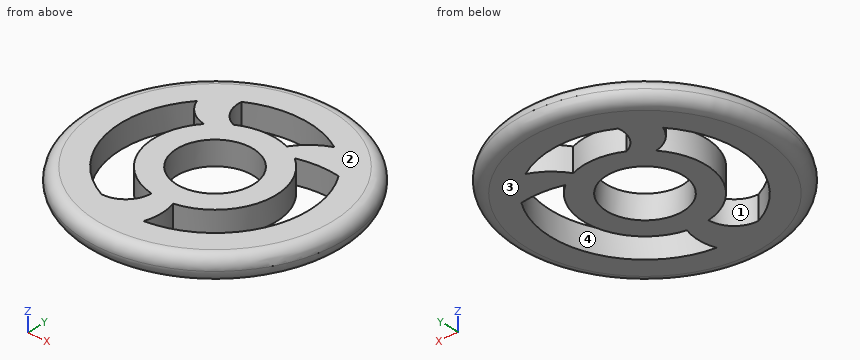
from build123d import *

# Parameters (mm, degrees)
F0_R     = 38.1945033512
F0_R_2   = 11.3
F1_DEPTH = 7
F2_R     = 3.49999


# Not quite as in the source:
# - a fillet or chamfer is up to 0.001 mm smaller than in the source, because OpenCascade refuses the exact size


with BuildPart() as f1:
    # F0 (on Top) → F1 (new body)
    with BuildSketch(Plane.XY):
        Circle(F0_R)
        with BuildLine():
            ThreePointArc((-11.1190587191, -25.3990096631), (-26.9847609568, -6.3691313979), (-21.3025923236, 17.7466255653))
            ThreePointArc((-21.3025923236, 17.7466255653), (-18.3465502514, 13.6852419499), (-13.7577746625, 11.6416763896))
            ThreePointArc((-13.7577746625, 11.6416763896), (-16.9304092047, -6.1778828887), (-3.0268251987, -17.7663536507))
            ThreePointArc((-3.0268251987, -17.7663536507), (-5.4906522747, -23.2602441725), (-11.1190587191, -25.3990096631))
        make_face(mode=Mode.SUBTRACT)
        with BuildLine():
            ThreePointArc((3.3689917925, -27.5207749339), (4.1908869079, -22.6127160748), (3.3689917925, -17.7046572157))
            ThreePointArc((3.3689917925, -17.7046572157), (17.5564618696, -4.0713191283), (10.8174583905, 14.4148391179))
            ThreePointArc((10.8174583905, 14.4148391179), (16.8916900663, 15.5906448864), (23.0748101796, 15.3719320138))
            ThreePointArc((23.0748101796, 15.3719320138), (25.1945379599, -11.5749045633), (3.3689917925, -27.5207749339))
        make_face(mode=Mode.SUBTRACT)
        Circle(F0_R_2, mode=Mode.SUBTRACT)
        with BuildLine():
            ThreePointArc((-8.6949064417, 15.7861836678), (-12.603803519, 19.1055384299), (-13.6713432148, 24.1213086993))
            ThreePointArc((-13.6713432148, 24.1213086993), (0.373914134, 27.7236964866), (14.3169083029, 23.7438264673))
            ThreePointArc((14.3169083029, 23.7438264673), (9.7472249081, 20.9497927504), (6.2279462514, 16.9120571875))
            ThreePointArc((6.2279462514, 16.9120571875), (-1.3558653844, 17.9712721276), (-8.6949064417, 15.7861836678))
        make_face(mode=Mode.SUBTRACT)
    extrude(amount=F1_DEPTH)

    # F2 (radius 3.5 in the source; OpenCascade refuses exactly that, so slightly less here)
    f2_edges = [f1.edges().sort_by_distance(p)[0] for p in [
        (-38.194503, 0, 7),
        (-38.194503, 0, 0),
    ]]
    fillet(f2_edges, radius=F2_R)


solid = f1.part
For this review, take the finished solid that the model builds, in its own axes (mm). Face numbers are marked on the shaded views. A direction names the side the tool comes from. Round coordinates to 2 decimals unless told otherwise and drop trailing zeros. Order: outer loops, then holes, each group sorted by start corner. A loop starts at its lowest first (then second) coordinate and runs counter-clockwise, first axis right, second up. Notation, with made-up numbers: M 77,50 L 114,50 A27 cw 114,85 Z; hole C 63,25 d4. An arc over 180 degrees is marked long. Use a Markdown table: item, result. Add a question column.
Item 1: To check wall thickness, follow line 1 along Y through (x, z) = (-6.5, 5); line 2 along X through (y, z) = (6, 1.75); line 3 along Y through (x, z) = (0, 5.25). State the ranges of each line that lie inside material, in increasing order.
Item 2: Tool access review of the marked faces 1 and 2: name each direction out of +Z, -Z, +X, -X, +Y, -Y from which nothing blocks a thin tool from reaching the whole face with its end or side.
Item 3: Mouldability with a two-part tool opening along Y and no side actions: class the marked faces 3 and 4 as released by +Y, released by -Y, zero draft, split by the parting line, or undercut.
Item 4: Insertion check: pin 1 (2 mm diameter, centred on x = -5, z = 3, fed in from -Y); pin 2 (20.5 mm diameter, centred on x = 0, y = 0, fed in from +Z); pin 3 (4 mm diameter, centred on y = 18.5, z = 3, fed in from +X); pin 4 (1.5 mm diameter, centred on y = 3, z = 3.5, fed in from -X). Each pin has a flat end and moves straight along its axis. Give the tip position at first contact, or say it passes through.
Item 5: Add section A-A, the plane x = 0. State how many separate pieces and enclosed holes the cut face has, then the cut area to 3 significant figures.
Item 6: Add section C-C, the plane z = 5.5. Give the boundary of the cut face in (x, y).
Geometry results:
| question | item | result |
|---|---|---|
| 1 | line 1 | y = -37.29 to -24.07, -16.81 to -9.24, 9.24 to 16.81, 26.95 to 37.29 |
| 1 | line 2 | x = -37.25 to -27.07, -16.99 to -9.58, 9.58 to 16.99, 27.07 to 37.25 |
| 1 | line 3 | y = -37.73 to -11.3, 11.3 to 18.02, 27.73 to 37.73 |
| 2 | face 1 | +Z, -Z |
| 2 | face 2 | +Z, +X, -X, +Y, -Y |
| 3 | face 3 | zero draft |
| 3 | face 4 | undercut |
| 4 | pin 1 | stops at y = -37.97 |
| 4 | pin 2 | passes through |
| 4 | pin 3 | stops at x = 34.43 |
| 4 | pin 4 | stops at x = -38.13 |
| 5 | separate pieces | 3 |
| 5 | enclosed holes | 0 |
| 5 | area | 298 mm² |
| 6 | outline | C 0,0 d75.13; hole M -21.3,17.75 A27.73 ccw -11.12,-25.4 A7.86 ccw -3.03,-17.77 A18.02 cw -13.76,11.64 A9.72 cw Z; hole M -13.67,24.12 A7.95 ccw -8.69,15.79 A18.02 cw 6.23,16.91 A17.62 cw 14.32,23.74 A27.73 ccw Z; hole C 0,0 d22.6; hole M 3.37,-27.52 A27.73 ccw 23.07,15.37 A27.37 ccw 10.82,14.41 A18.02 cw 3.37,-17.7 A15.07 cw Z |
